For this review, use the dimensioned drawing (mm, ordinates from the lowest corner) and the shaded views. Coordinates: 2 decimals unless noted, no trailing zeros. Loops run counter-clockwise (first coordinate to the right, second up) from the corner with the lowest first, then second, coordinate; pieces in that order, holes last.
1. Take a section at B-B, the plane x = 1.75. Count the separate pieces of the cut face and the enclosed holes in it, then the cut area to 3 significant figures.
2. Clearance check with flat-ended pins moving along their axes: P1, Ø5, axis at y = 25, z = 77.5, coming from the +X side; P2, Ø2, axis at x = 4.5, y = 19, coming from the +Z side; P3, Ø4, axis at x = 3, z = 49.5, coming from the +Y side (1 decimal); P4, Ø1, axis at x = 2, z = 38.5, coming from the -Y side. State where each tip first meets the part, or that it passes through.
3. Take a section at A-A, the plane z = 42.5. State the section outline as (x, y) points.
4. Mouldability with a two-part tool opening along Z and no side actions: class the marked faces 1, 2 and 3 as pulls with the +Z half, pulls with the -Z half, needs draft (parallel to the pull), parting line crosses it, or undercut.
5. Take a section at D-D, the plane y = 25. State the section outline as (x, z) points, then the cut area to 3 significant figures.
6. To check wall thickness, follow probe 1 along Y at (x, z) = (1.75, 42.5); probe 2 along Z at (x, y) = (7.5, 21.5) (1 decimal); probe 3 along Y at (x, z) = (1.5, 7.5). State the ranges of each line that lie inside material, in increasing order.
7. Take a section at C-C, the plane y = 11. State the section outline as (x, z) points, then the cut area to 3 significant figures.
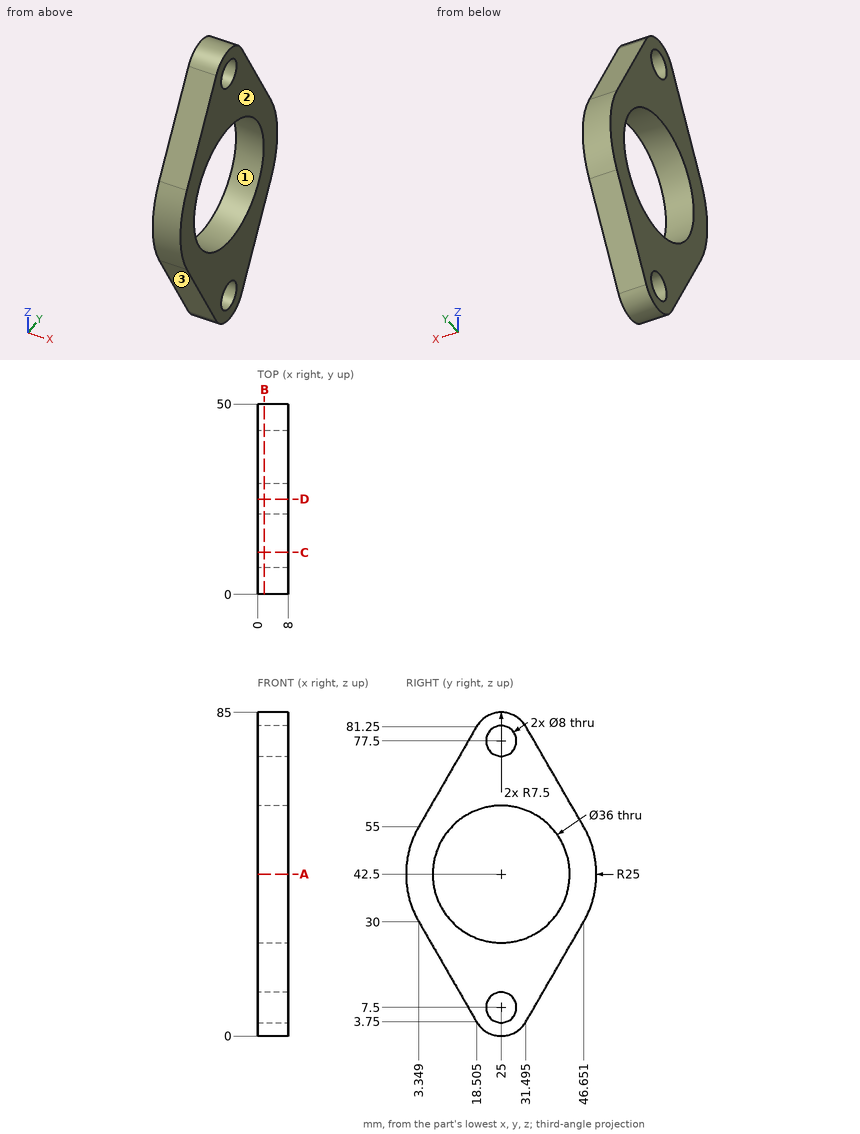
Results list:
1. separate pieces: 1
1. enclosed holes: 3
1. area: 1,620 mm2
2. P1: passes through
2. P2: stops at z = 83.09
2. P3: stops at y = 49.5
2. P4: stops at y = 0.25
3. outline: (0, 0) - (8, 0) - (8, 7) - (0, 7) - close; (0, 43) - (8, 43) - (8, 50) - (0, 50) - close
4. face 1: undercut
4. face 2: needs draft
4. face 3: pulls with the -Z half
5. outline: (0, 0) - (8, 0) - (8, 3.5) - (0, 3.5) - close; (0, 11.5) - (8, 11.5) - (8, 24.5) - (0, 24.5) - close; (0, 60.5) - (8, 60.5) - (8, 73.5) - (0, 73.5) - close; (0, 81.5) - (8, 81.5) - (8, 85) - (0, 85) - close
5. area: 264 mm2
6. probe 1: y = 0 to 7, 43 to 50
6. probe 2: z = 0.9 to 5.6, 9.4 to 24.8, 60.2 to 75.6, 79.4 to 84.1
6. probe 3: y = 16.34 to 21, 29 to 33.66
7. outline: (0, 16.75) - (8, 16.75) - (8, 31.19) - (0, 31.19) - close; (0, 53.81) - (8, 53.81) - (8, 68.25) - (0, 68.25) - close
7. area: 231 mm2
